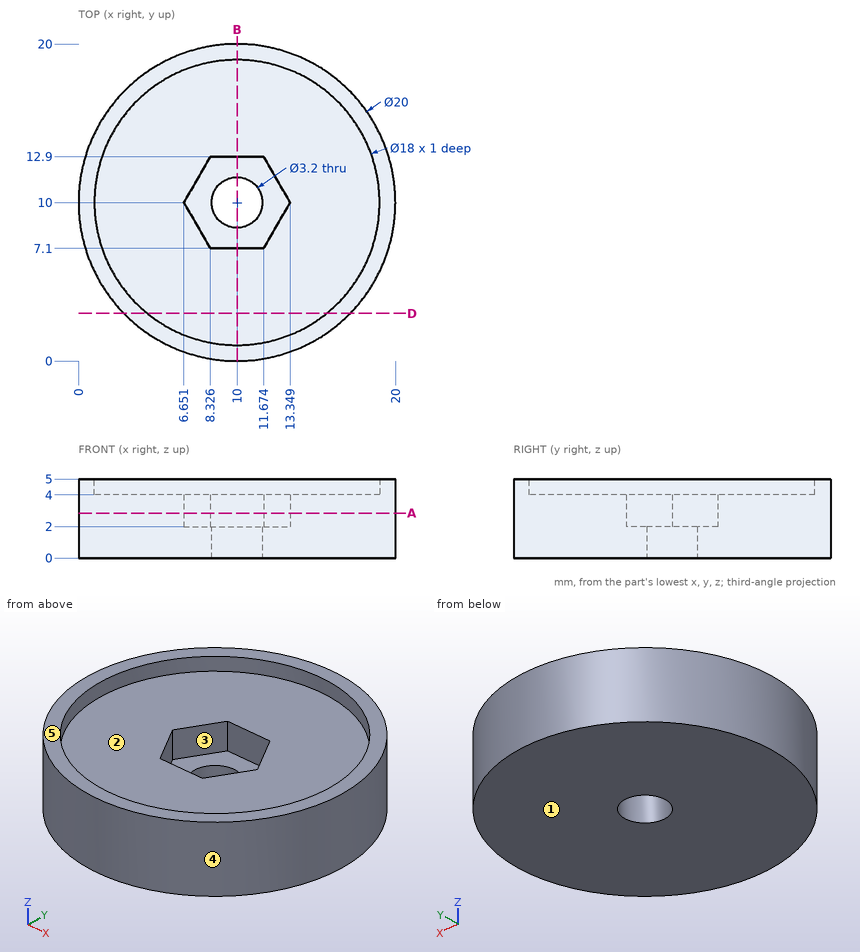
Can you work these out from the drawing? Everything is in mm from the part's minimum corner. A direction names the side the tool comes from. Coordinates: 2 decimals unless noted, no trailing zeros. Loops run counter-clockwise (first coordinate to the right, second up) from the corner with the lowest first, then second, coordinate; pieces in that order, holes last. Notation, with made-up numbers: (-7.75, -34.75) - (35.25, -34.75) arc R29 cw to (35.25, -6.75) - close; hole circle Ø7 at (-26.5, -12.75). An arc over 180 degrees is marked (long way). Put each result on its own line as item: value. Start each with the question number.
Item 1: Which directions (+Z, -Z, +X, -X, +Y, -Y) give clear straight access to the entire face, cutting with the end or side of a thin tool? Please do the marked faces 1 and 2.
Item 2: Suppose I cut it at A-A (z = 2.85). Please give me the cut outline in (x, y) (1 decimal), and give its area (3 significant figures).
Item 3: If we mould it in two halves opening along Y, with no side actions, what happens to the marked faces 3, 4 and 5? For each: +Y half, -Y half, draft (parallel to the pull), parting line (faces both ways), or undercut.
Item 4: If I drill on line 1 along Y through (x, z) = (10, 4.5); line 2 along Y through (x, z) = (10, 0.95); line 3 along Z through (x, y) = (13.5, 14.5), over which ranges is the centre line in solid material (lowest first)?
Item 5: Suppose I cut it at B-B (x = 10). Please give me the cut outline in (y, z), and give its area (3 significant figures).
Item 6: Suppose I cut it at D-D (y = 3). Please give me the cut outline in (x, z), and give its area (3 significant figures).
Item 7: For pin 1 (5 mm diameter, centred on x = 7, y = 4.5, fed in from +Z); pin 2 (2 mm diameter, centred on y = 9, z = 3, fed in from +X); pin 3 (3 mm diameter, centred on x = 10, y = 10, fed in from +Z); pin 4 (1 mm diameter, centred on y = 15, z = 0.5, fed in from +X), each with a flat end and sliding along its axis, tell me the tip position at first contact or that it passes through.
Here are the results:
1. face 1: -Z, +X, -X, +Y, -Y
1. face 2: +Z
2. outline: circle Ø20 at (10, 10); hole (6.7, 10) - (8.3, 7.1) - (11.7, 7.1) - (13.3, 10) - (11.7, 12.9) - (8.3, 12.9) - close
2. area: 285 mm²
3. face 3: undercut
3. face 4: parting line
3. face 5: draft
4. line 1: 0 to 1, 19 to 20
4. line 2: 0 to 8.4, 11.6 to 20
4. line 3: 0 to 4
5. outline: (0, 0) - (8.4, 0) - (8.4, 2) - (7.1, 2) - (7.1, 4) - (1, 4) - (1, 5) - (0, 5) - close; (11.6, 0) - (20, 0) - (20, 5) - (19, 5) - (19, 4) - (12.9, 4) - (12.9, 2) - (11.6, 2) - close
5. area: 64.0 mm²
6. outline: (2.86, 0) - (17.14, 0) - (17.14, 5) - (15.66, 5) - (15.66, 4) - (4.34, 4) - (4.34, 5) - (2.86, 5) - close
6. area: 60.1 mm²
7. pin 1: z = 4
7. pin 2: x = 20
7. pin 3: through
7. pin 4: x = 18.93
